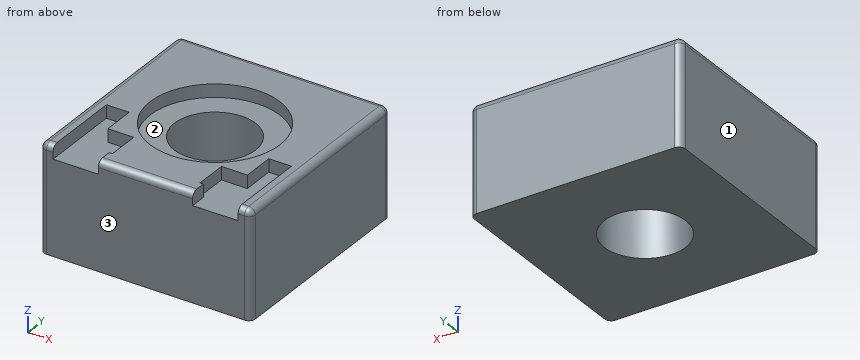
from build123d import *

# Parameters (mm, degrees)
SKETCH_W        = 6.5
SKETCH_H        = 6.5
PAD_DEPTH       = 3.3
SKETCH001_R     = 1.25
POCKET_DEPTH    = 3.3
SKETCH002_R     = 2
POCKET001_DEPTH = 0.4
FILLET_R        = 0.2


with BuildPart() as part:
    # Sketch → Pad (new body)
    with BuildSketch(Plane.XY):
        Rectangle(SKETCH_W, SKETCH_H)
    extrude(amount=PAD_DEPTH)

    # Sketch001 (on Face6 of Pad) → Pocket (cut)
    with BuildSketch(Plane.XY.offset(3.3)):
        Circle(SKETCH001_R)
    extrude(amount=-POCKET_DEPTH, mode=Mode.SUBTRACT)

    # Sketch002 (on Face5 of Pocket) → Pocket001 (cut)
    with BuildSketch(Plane.XY.offset(3.3)):
        Circle(SKETCH002_R)
        Polygon((-2.85, -0.75), (-2.15, -0.75), (-2.15, -1.75), (-1.35, -1.75), (-1.35, -2.75), (-1.45, -2.75), (-1.45, -3.25), (-2.85, -3.25), align=None)
        Polygon((2.15, -0.75), (2.85, -0.75), (2.85, -3.25), (1.45, -3.25), (1.45, -2.75), (1.35, -2.75), (1.35, -1.75), (2.15, -1.75), align=None)
    extrude(amount=-POCKET001_DEPTH, mode=Mode.SUBTRACT)

    # Fillet
    fillet_edges = [part.edges().sort_by_distance(p)[0] for p in [
        (-3.25, -3.25, 1.65),
        (3.25, -3.25, 1.65),
        (3.25, 3.25, 1.65),
        (-3.25, 3.25, 1.65),
        (0, -3.25, 3.3),
        (-3.05, -3.25, 3.3),
        (3.05, -3.25, 3.3),
        (3.25, 0, 3.3),
        (-3.25, 0, 3.3),
        (0, 3.25, 3.3),
    ]]
    fillet(fillet_edges, radius=FILLET_R)


solid = part.part
Geometry check sheet. Reference: the model listing, model coordinates, mm. Face numbers are marked on the shaded views. Round coordinates to 2 decimals unless told otherwise and drop trailing zeros. Order: outer loops, then holes, each group sorted by start corner. A loop starts at its lowest first (then second) coordinate and runs counter-clockwise, first axis right, second up. Notation, with made-up numbers: M 29,15.25 L 64,15.25 A25 cw 64,33.25 Z; hole C 85,-6 d4. An arc over 180 degrees is marked long. Write each question's results on one line, items separated by ' | '. Start each with the question number.
1. Cross-section at C-C on z = 0.3. Record the boundary of the cut face in (x, y).
2. Draft check along X on the marked faces 1, 2 and 3. Enter one of: pulls with the +X half, pulls with the -X half, needs draft (parallel to the pull), parting line crosses it, or undercut.
3. Cross-section at D-D on y = -2.5. Record the boundary of the cut face in (x, z).
4. Go/stop test with a flat-tipped pin: P1, Ø0.8, axis at x = -2, y = -2.5, coming from the +Z side. Record where the tip stops, or that it passes through.
5. Cross-section at A-A on y = 0. Record the boundary of the cut face in (x, z), plus the area to 3 significant figures.
6. Material ranges on L1, parallel to Y at x = 0, z = 3; L2, parallel to Y at x = 0, z = 0.75; L3, parallel to Z at x = 0.5, y = -1.5, recorded low to high. Write a range as from..to.
Resolved:
1) outline: M -3.25,-3.05 A0.2 ccw -3.05,-3.25 L 3.05,-3.25 A0.2 ccw 3.25,-3.05 L 3.25,3.05 A0.2 ccw 3.05,3.25 L -3.05,3.25 A0.2 ccw -3.25,3.05 Z; hole C 0,0 d2.5
2) face 1: pulls with the -X half | face 2: undercut | face 3: needs draft
3) outline: M -3.25,0 L 3.25,0 L 3.25,3.1 A0.2 ccw 3.05,3.3 L 2.85,3.3 L 2.85,2.9 L 1.35,2.9 L 1.35,3.3 L -1.35,3.3 L -1.35,2.9 L -2.85,2.9 L -2.85,3.3 L -3.05,3.3 A0.2 ccw -3.25,3.1 Z
4) P1: z = 2.9
5) outline: M -3.25,0 L -1.25,0 L -1.25,2.9 L -2,2.9 L -2,3.3 L -3.05,3.3 A0.2 ccw -3.25,3.1 Z; M 1.25,0 L 3.25,0 L 3.25,3.1 A0.2 ccw 3.05,3.3 L 2,3.3 L 2,2.9 L 1.25,2.9 Z | area: 12.6 mm2
6) L1: -3.25..-2, 2..3.25 | L2: -3.25..-1.25, 1.25..3.25 | L3: 0..2.9
